```python
from build123d import *

# Parameters (mm, degrees)
CROQUIS1_R              = 12.5
SALIENTE_EXTRUIR1_DEPTH = 1.5
CROQUIS2_R              = 0.75
CROQUIS4_R              = 10
CORTAR_EXTRUIR1_DEPTH   = 18.930421077


with BuildPart() as part:
    # Croquis1 → Saliente-Extruir1 (new, symmetric)
    with BuildSketch(Plane(origin=(0, 0, 0), x_dir=(1, 0, 0), z_dir=(0, 1, 0))):
        with Locations(Location((0, 0, 0), (0, 0, 270))):
            Circle(CROQUIS1_R)
    extrude(amount=SALIENTE_EXTRUIR1_DEPTH, both=True)

    # Croquis2 → Cortar-Revolución1 (revolve, cut)
    with BuildSketch(Plane(origin=(0, 0, 0), x_dir=(0, 0, -1), z_dir=(1, 0, 0)), mode=Mode.PRIVATE) as cortar_revoluci_n1_sk:
        with Locations((12.5, 0)):
            Circle(CROQUIS2_R)
    revolve(cortar_revoluci_n1_sk.sketch.rotate(Axis((0, 1.5, 0), (0, -1, 0)), 180), axis=Axis((0, 1.5, 0), (0, -1, 0)), mode=Mode.SUBTRACT)

    # Croquis4 → Cortar-Extruir1 (cut, through all)
    with BuildSketch(Plane.XZ.offset(1.5)):
        with Locations(Location((0, 0, 0), (0, 0, 270))):
            Circle(CROQUIS4_R)
    extrude(amount=-CORTAR_EXTRUIR1_DEPTH, mode=Mode.SUBTRACT)


solid = part.part
```
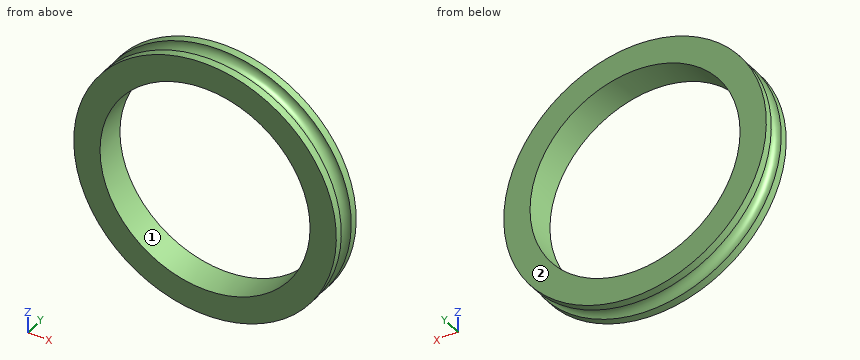
Build history of the part. All positions in model axes, mm. Face numbers are marked on the shaded views. Round coordinates to 2 decimals unless told otherwise and drop trailing zeros. Order: outer loops, then holes, each group sorted by start corner. A loop starts at its lowest first (then second) coordinate and runs counter-clockwise, first axis right, second up. Notation, with made-up numbers: (69, -2.75) - (124, -2.75) arc R23 cw to (124, 20.25) - close; hole circle Ø3 at (4, 19.5). An arc over 180 degrees is marked (long way). Use a Markdown table: item, result.
1) Saw through at C-C on y = 0. Write the cut outline in (x, z).
Recorded:
| item | result |
|---|---|
| outline | circle Ø23.5 at (0, 0); hole circle Ø20 at (0, 0) |
2) Saw through at A-A on x = 0. Write the cut outline in (y, z), and give its area (3 significant figures).
Recorded:
| item | result |
|---|---|
| outline | (-1.5, -12.5) - (-0.75, -12.5) arc R0.75 cw to (0.75, -12.5) - (1.5, -12.5) - (1.5, -10) - (-1.5, -10) - close; (-1.5, 10) - (1.5, 10) - (1.5, 12.5) - (0.75, 12.5) arc R0.75 cw to (-0.75, 12.5) - (-1.5, 12.5) - close |
| area | 13.2 mm² |
3) Pull direction X, two halves, no side cores. Call the marked faces 1 and 2: pulls with the +X half, pulls with the -X half, needs draft (parallel to the pull), parting line crosses it, or undercut.
Recorded:
| item | result |
|---|---|
| face 1 | undercut |
| face 2 | needs draft |
4) Flat gauge pins, fed straight in: pin 1 Ø1 at (y, z) = (0.5, 9) entering from -X; pin 2 Ø1 at (x, y) = (3.5, -0.5) entering from -Z. Where does each tip first touch, or does it go through?
Recorded:
| item | result |
|---|---|
| pin 1 | stops at x = -9.1 |
| pin 2 | stops at z = -12.12 |
5) Saw through at B-B on z = 0. Write the cut outline in (x, y).
Recorded:
| item | result |
|---|---|
| outline | (-12.5, -1.5) - (-10, -1.5) - (-10, 1.5) - (-12.5, 1.5) - (-12.5, 0.75) arc R0.75 cw to (-12.5, -0.75) - close; (10, -1.5) - (12.5, -1.5) - (12.5, -0.75) arc R0.75 cw to (12.5, 0.75) - (12.5, 1.5) - (10, 1.5) - close |
6) Wall check: L1, parallel to X at y = 0.95, z = 0; L2, parallel to Z at x = 7, y = 1.2; L3, parallel to X at y = -0.15, z = 0. Give the ranges that are in metal, low to high.
Recorded:
| item | result |
|---|---|
| L1 | x = -12.5 to -10, 10 to 12.5 |
| L2 | z = -10.36 to -7.14, 7.14 to 10.36 |
| L3 | x = -11.77 to -10, 10 to 11.77 |
